Verification items for the finished model (mm, model axes). Face numbers are marked on the shaded views. A direction names the side the tool comes from. Give positions to 0.01 mm unless a question says otherwise; leave off trailing zeros. Order: outer loops, then holes, each group sorted by start corner. A loop starts at its lowest first (then second) coordinate and runs counter-clockwise, first axis right, second up. Notation, with made-up numbers: (-15.75, 50) - (-6.75, 50) arc R22 ccw to (-6.75, 89) - close; hole circle Ø9 at (80.25, -30). An arc over 180 degrees is marked (long way). Answer as a JSON object with one key per item and string values.
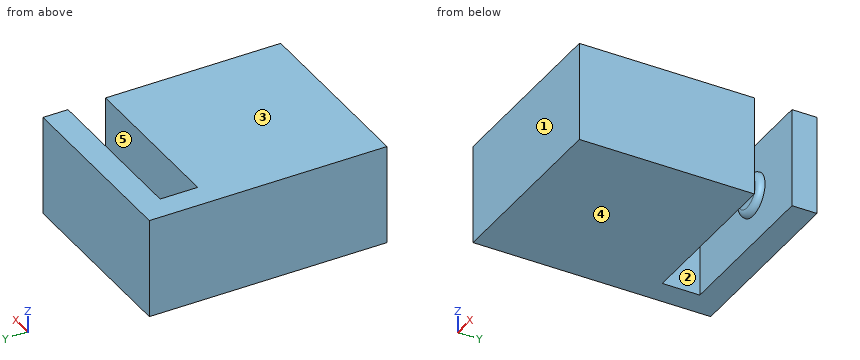
```python
from build123d import *

# Parameters (mm, degrees)
F1_DEPTH = 8
F2_R     = 1.7
F3_DEPTH = 0.5
F4_R     = 0.49999


# Not quite as in the source:
# - a fillet or chamfer is up to 0.001 mm smaller than in the source, because OpenCascade refuses the exact size


with BuildPart() as f1:
    # F0 (on Top) → F1 (new body)
    with BuildSketch(Plane.XY):
        Polygon((-7.5, -9.5), (7.5, -9.5), (7.5, 4.5), (-5.5, 4.5), (-5.5, 7.5), (7.5, 7.5), (7.5, 9.5), (-7.5, 9.5), align=None)
    extrude(amount=F1_DEPTH)

    # F2 (on face) → F3 (join)
    with BuildSketch(Plane.XZ.offset(-7.5)):
        with Locations((2, 4)):
            Circle(F2_R)
    extrude(amount=F3_DEPTH)

    # F4 (radius 0.5 in the source; OpenCascade refuses exactly that, so slightly less here)
    f4_edges = [f1.edges().sort_by_distance(p)[0] for p in [
        (0.3, 7, 4),
    ]]
    fillet(f4_edges, radius=F4_R)


solid = f1.part
```
(1) Access from +Z, -Z, +X, -X, +Y, -Y to the whole of each face (thin tool, end or side, straight path). Record for the marked faces 4 and 5.
Computed values:
{"face 4": "-Z, +X, -X, +Y, -Y", "face 5": "+Z, -Z, +X"}
(2) Section check C-C (x = 4). Record the cut outline in (y, z).
Computed values:
{"outline": "(-9.5, 0) - (4.5, 0) - (4.5, 8) - (-9.5, 8) - close; (7.5, 0) - (9.5, 0) - (9.5, 8) - (7.5, 8) - close"}
(3) Release check for a two-part mould opening along Y. For the marked faces 1, 2 and 3 record: pulls with the +Y half, pulls with the -Y half, needs draft (parallel to the pull), parting line crosses it, or undercut.
Computed values:
{"face 1": "pulls with the -Y half", "face 2": "undercut", "face 3": "needs draft"}
(4) Material ranges on line 1 along Y through (x, z) = (5, 5.25); line 2 along Y through (x, z) = (1.5, 3.75); line 3 along X through (y, z) = (6.5, 5.75), recorded low to high. Write a range as [from, to].
Computed values:
{"line 1": "y = [-9.5, 4.5], [7.5, 9.5]", "line 2": "y = [-9.5, 4.5], [7, 9.5]", "line 3": "x = [-7.5, -5.5]"}
(5) Section check D-D (y = 5.5). Record the cut outline in (x, z).
Computed values:
{"outline": "(-7.5, 0) - (-5.5, 0) - (-5.5, 8) - (-7.5, 8) - close"}
(6) Gauge pin test, flat end, axial feed: pin 1 Ø1.5 at (y, z) = (6, 5) entering from +X. Record the tip position at first contact, or that the pin passes through.
Computed values:
{"pin 1": "stops at x = -5.5"}
